The drawing under review shows one solid part. Ordinate dimensions are in mm from its lowest x, y, z. A direction names the side the tool comes from. Coordinates: 2 decimals unless noted, no trailing zeros. Write each loop counter-clockwise with the first axis right and the second up, starting at its lowest first coordinate (ties: lowest second). Pieces come first, ordered by that corner, then holes. Notation, with made-up numbers: (-23, -19) - (23, -19) arc R12 ccw to (23, -7) - close; hole circle Ø8 at (84.25, -7.75). An arc over 180 degrees is marked (long way). Use a Markdown table: item, result.
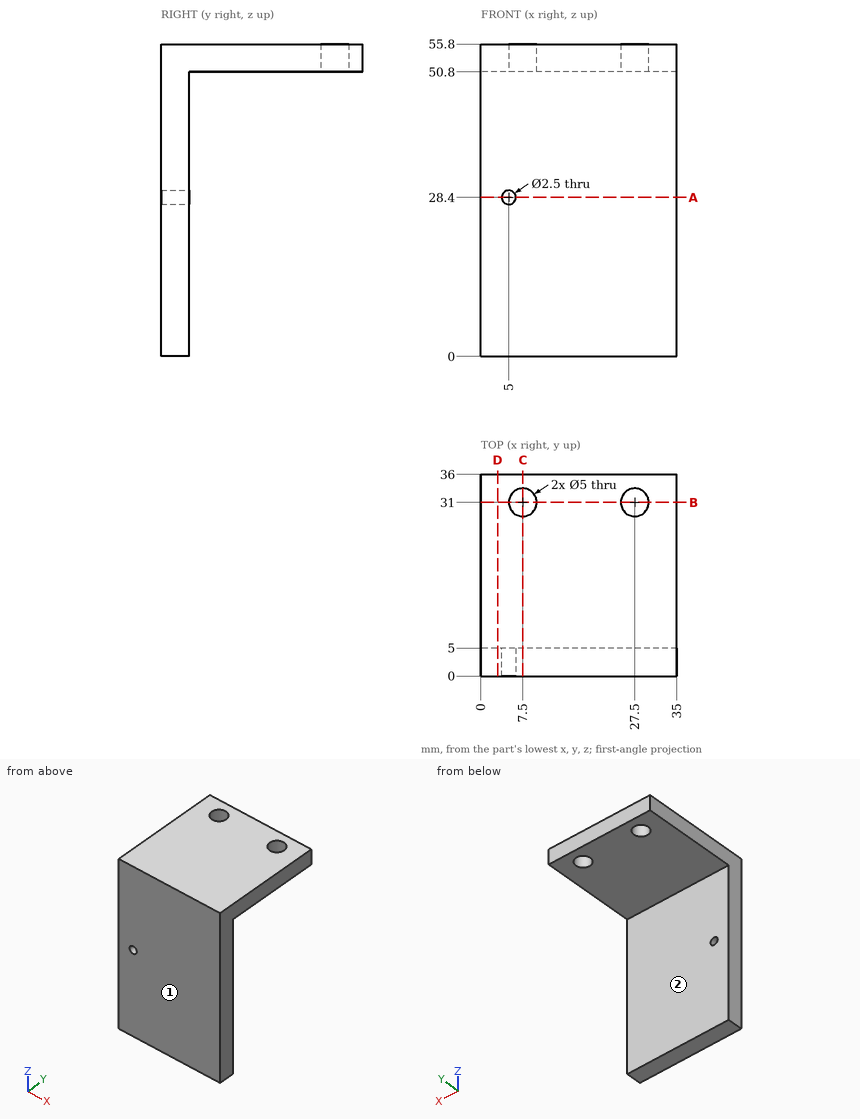
(1) Take a section at B-B on y = 31. Write out the cut boundary in (x, z), and give its area (3 significant figures).
Determined:
| item | result |
|---|---|
| outline | (0, 50.8) - (5, 50.8) - (5, 55.8) - (0, 55.8) - close; (10, 50.8) - (25, 50.8) - (25, 55.8) - (10, 55.8) - close; (30, 50.8) - (35, 50.8) - (35, 55.8) - (30, 55.8) - close |
| area | 125 mm2 |
(2) Take a section at C-C on x = 7.5. Write out the cut boundary in (y, z).
Determined:
| item | result |
|---|---|
| outline | (0, 0) - (5, 0) - (5, 50.8) - (28.5, 50.8) - (28.5, 55.8) - (0, 55.8) - close; (33.5, 50.8) - (36, 50.8) - (36, 55.8) - (33.5, 55.8) - close |
(3) Take a section at A-A on z = 28.4. Write out the cut boundary in (x, y), and give its area (4 significant figures).
Determined:
| item | result |
|---|---|
| outline | (0, 0) - (3.75, 0) - (3.75, 5) - (0, 5) - close; (6.25, 0) - (35, 0) - (35, 5) - (6.25, 5) - close |
| area | 162.5 mm2 |
(4) Machinability: for the marked faces 1 and 2, which of the approach directions +Z, -Z, +X, -X, +Y, -Y give a long, thin tool a straight path to every point of the face, cutting with its end or side? Answer none if there is none.
Determined:
| item | result |
|---|---|
| face 1 | +Z, -Z, +X, -X, -Y |
| face 2 | -Z, +X, -X, +Y |
(5) Take a section at D-D on x = 3. Write out the cut boundary in (y, z).
Determined:
| item | result |
|---|---|
| outline | (0, 0) - (5, 0) - (5, 50.8) - (36, 50.8) - (36, 55.8) - (0, 55.8) - close |
(6) For pin 1 (10.5 mm diameter, centred on x = 20, z = 37.5, fed in from +Y), flat-tipped, find the tip position at first contact; note if it passes through.
Determined:
| item | result |
|---|---|
| pin 1 | y = 5 |
(7) For L1, parallel to Z at x = 5, y = 3.4; L2, parallel to X at y = 2.7, z = 28.4; L3, parallel to Y at x = 27.5, z = 52.55, list the stretches that pass through material, from the lowest coordinate up. Write a range as from..to.
Determined:
| item | result |
|---|---|
| L1 | 0..27.15, 29.65..55.8 |
| L2 | 0..3.75, 6.25..35 |
| L3 | 0..28.5, 33.5..36 |
